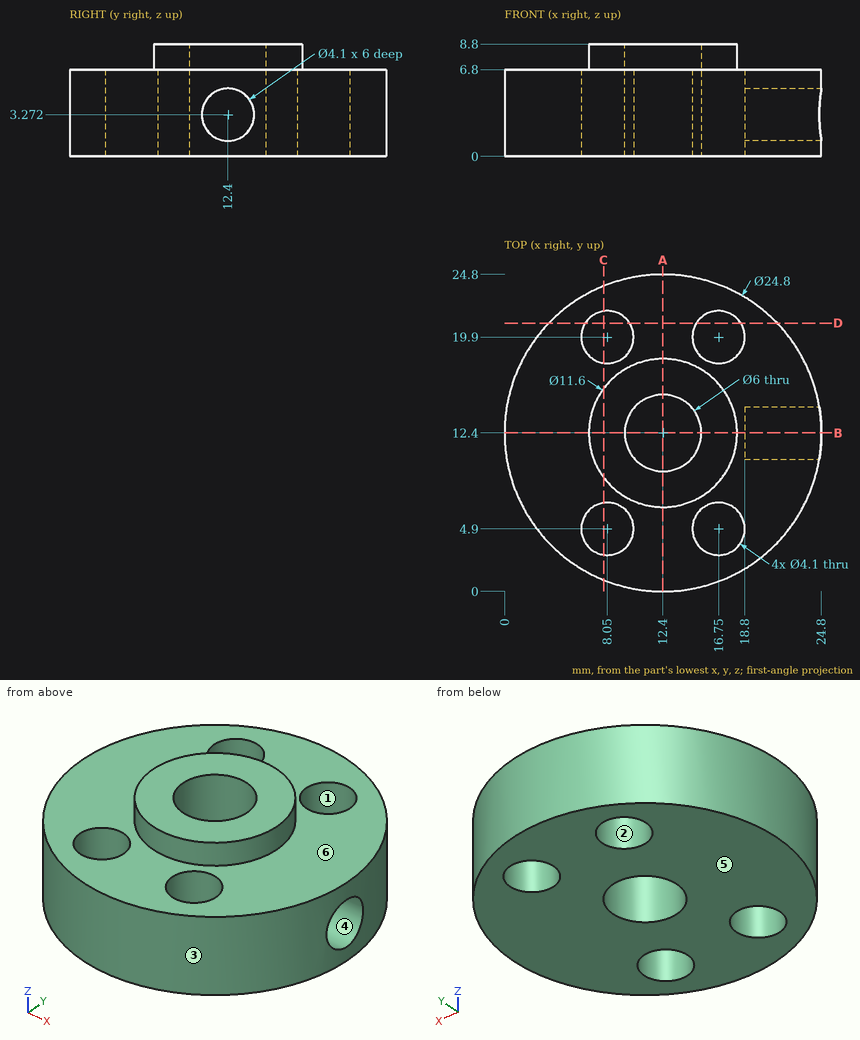
Could you check a few things on this drawing? It's one solid part, dimensions in mm from its lowest x, y, z. A direction names the side the tool comes from. Round coordinates to 2 decimals unless told otherwise and drop trailing zeros. Loops run counter-clockwise (first coordinate to the right, second up) from the corner with the lowest first, then second, coordinate; pieces in that order, holes last.
Q1. Please list where these lines run through material, in increasing order: L1, parallel to X at y = 6.75, z = 1.5; L2, parallel to X at y = 21.5, z = 4.5; L3, parallel to Y at x = 16.5, z = 1 (1 decimal).
Q2. I want a section at B-B (y = 12.4). Write out the boundary of the cut face in (x, z), and give its area (3 significant figures).
Q3. I want a section at D-D (y = 21). Write out the boundary of the cut face in (x, z).
Q4. I want a section at C-C (x = 7.75). Write out the boundary of the cut face in (y, z) (1 decimal).
Q5. On a 3-axis mill with a long thin cutter (end or side, diameter ignored), from which of +Z, -Z, +X, -X, +Y, -Y can I reach the whole of each face in a straight line? I mean the marked faces 5 and 6. Say none if no direction works.
Q6. For P1, Ø4, axis at y = 8, z = 7.5, coming from the +X side; P2, Ø5, axis at x = 21, z = 6, coming from the -Y side; P3, Ø3.5, axis at y = 12.4, z = 3.27, coming from the +X side; P4, Ø5.5, axis at x = 16.75, y = 4.9, coming from the -Z side, each with a flat end and sliding along its axis, tell me the tip position at first contact or that it passes through.
Q7. I want a section at A-A (x = 12.4). Write out the boundary of the cut face in (y, z).
Q8. Thinking about a two-plate mould opening in X: for the marked faces 1, 2, 3 and 4, which applies, pulls with the +X half, pulls with the -X half, needs draft (parallel to the pull), parting line crosses it, or undercut?
Answer below:
1. L1: x = 1.36 to 7.17, 8.93 to 15.87, 17.63 to 23.44
1. L2: x = 3.98 to 6.77, 9.33 to 15.47, 18.03 to 20.82
1. L3: y = 0.7 to 2.9, 6.9 to 17.9, 21.9 to 24.1
2. outline: (0, 0) - (9.4, 0) - (9.4, 8.8) - (6.6, 8.8) - (6.6, 6.8) - (0, 6.8) - close; (15.4, 0) - (24.8, 0) - (24.8, 1.22) - (18.8, 1.22) - (18.8, 5.32) - (24.8, 5.32) - (24.8, 6.8) - (18.2, 6.8) - (18.2, 8.8) - (15.4, 8.8) - close
2. area: 114 mm2
3. outline: (3.47, 0) - (6.32, 0) - (6.32, 6.8) - (3.47, 6.8) - close; (9.78, 0) - (15.02, 0) - (15.02, 6.8) - (9.78, 6.8) - close; (18.48, 0) - (21.33, 0) - (21.33, 6.8) - (18.48, 6.8) - close
4. outline: (0.9, 0) - (2.9, 0) - (2.9, 6.8) - (0.9, 6.8) - close; (6.9, 0) - (17.9, 0) - (17.9, 6.8) - (15.9, 6.8) - (15.9, 8.8) - (8.9, 8.8) - (8.9, 6.8) - (6.9, 6.8) - close; (21.9, 0) - (23.9, 0) - (23.9, 6.8) - (21.9, 6.8) - close
5. face 5: -Z, +X, -X, +Y, -Y
5. face 6: +Z
6. P1: stops at x = 24.54
6. P2: stops at y = 1.6
6. P3: stops at x = 18.8
6. P4: stops at z = 0
7. outline: (0, 0) - (9.4, 0) - (9.4, 8.8) - (6.6, 8.8) - (6.6, 6.8) - (0, 6.8) - close; (15.4, 0) - (24.8, 0) - (24.8, 6.8) - (18.2, 6.8) - (18.2, 8.8) - (15.4, 8.8) - close
8. face 1: undercut
8. face 2: undercut
8. face 3: parting line crosses it
8. face 4: needs draft
